from build123d import *

# Parameters (mm, degrees)
F1_DEPTH = 63.5
F2_DEPTH = 7.9375
F3_DEPTH = 25.4
F0_W     = 25.4
F0_H     = 28.575
F5_R     = 6.35


with BuildPart() as f1:
    # F0 (on Front) → F1 (new body, symmetric)
    with BuildSketch(Plane.XZ):
        Polygon((41.275, -9.525), (41.275, 9.525), (22.225, 9.525), (-41.275, 9.525), (-41.275, -9.525), align=None)
    extrude(amount=F1_DEPTH, both=True)

    # F0 (on Front) → F2 (join, symmetric)
    with BuildSketch(Plane.XZ):
        with BuildLine():
            Line((-41.275, 9.525), (22.225, 9.525))
            Line((22.225, 9.525), (22.225, 27.673652))
            ThreePointArc((22.225, 27.673652), (30.148747, 49.82513), (50.324526, 61.9252))
            add(Edge.make_bspline(
                [(-41.275, 9.525), (-34.773878, 42.640614), (12.253828, 61.712361), (50.324526, 61.9252)],
                knots=[0, 0, 0, 0, 105.528452, 105.528452, 105.528452, 105.528452], degree=3))
        make_face()
    extrude(amount=F2_DEPTH, both=True)

    # F0 (on Front) → F3 (join, symmetric)
    with BuildSketch(Plane.XZ):
        with BuildLine():
            Line((22.225, 9.525), (41.275, 9.525))
            Line((41.275, 9.525), (41.275, 27.673652))
            ThreePointArc((41.275, 27.673652), (47.109768, 39.970374), (60.325, 43.227912))
            Line((60.325, 43.227912), (60.325, 61.9252))
            Line((60.325, 61.9252), (50.324526, 61.9252))
            ThreePointArc((50.324526, 61.9252), (30.148747, 49.82513), (22.225, 27.673652))
            Line((22.225, 27.673652), (22.225, 9.525))
        make_face()
        with BuildLine():
            Line((60.325, 61.9252), (60.325, 43.227912))
            ThreePointArc((60.325, 43.227912), (61.028899, 43.067475), (61.724775, 42.8752))
            Line((61.724775, 42.8752), (68.150982, 42.8752))
            Line((68.150982, 42.8752), (68.150982, 61.9252))
            Line((68.150982, 61.9252), (60.325, 61.9252))
        make_face()
    extrude(amount=F3_DEPTH, both=True)

    # F0 (on Front) → F4 (revolve)
    with BuildSketch(Plane.XZ):
        with Locations((98.425, 52.3875)):
            Rectangle(F0_W, F0_H)
    revolve(axis=Axis((85.725, 0, 52.3875), (0, 0, -1)))

    # F5
    f5_edges = [f1.edges().sort_by_distance(p)[0] for p in [
        (41.275, -63.5, 0),
        (-41.275, -63.5, 0),
        (41.275, 63.5, 0),
        (-41.275, 63.5, 0),
    ]]
    fillet(f5_edges, radius=F5_R)


solid = f1.part
Read the model definition and answer for the solid it produces. Units are mm, in the model's axes. A direction names the side the tool comes from. Round coordinates to 2 decimals unless told otherwise and drop trailing zeros. Write each loop counter-clockwise with the first axis right and the second up, starting at its lowest first coordinate (ties: lowest second). Pieces come first, ordered by that corner, then holes.
Q1. A tool of negligible diameter and unlimited length cuts with its end or side. For faces 5 (the face through (30.36, 16.55, 50.08)), 6 (the face through (40, -25.4, 36)), 7 (the face through (86, 0, 38.1)), 8 (the face through (0, -63.5, 0)), 9 (the face through (-6, -7.938, 30)), from which of +Z, -Z, +X, -X, +Y, -Y can it reach the whole face along a straight path? Write none if from no direction.
Values:
face 5: +Z, -X, +Y
face 6: +Z, +X, -X, -Y
face 7: -Z, +X, +Y, -Y
face 8: +Z, -Z, +X, -X, -Y
face 9: +Z, -X, -Y
Q2. The mould has two halves that part along X. Classify faces 1 (the face through (39.464, -61.59, 0.133)), 2 (the face through (57, 0, 61.925)), 3 (the face through (64, 19, 42.875)), 4 (the face through (22.225, -17, 19)): released by +X, released by -X, zero draft, split by the parting line, or undercut.
Values:
face 1: released by +X
face 2: zero draft
face 3: undercut
face 4: released by -X
Q3. Flat-ended cylindrical pins translate along their axes: P1, Ø1.5, axis at x = -13, z = 43.5, coming from the -Y side; P2, Ø1, axis at y = -18.5, z = 49.5, coming from the -X side; P3, Ø2, axis at x = -18.5, y = -43.5, coming from the +Z side (3 decimals). Find the tip coordinate at first contact, or state that the pin passes through.
Values:
P1: stops at y = -7.94
P2: stops at x = 29.49
P3: stops at z = 9.525
Q4. Find section A-A on y = -28. Determine the outline of the cut face in (x, z) (3 decimals), and give its area (3 significant figures).
Values:
outline: (-41.275, -9.525) - (41.275, -9.525) - (41.275, 9.525) - (-41.275, 9.525) - close
area: 1,570 mm2
Q5. Straight lines are drawn through the part: line 1 (Y direction, x = 22, z = 25); line 2 (X direction, y = -50.5, z = 4) (3 decimals); line 3 (Y direction, x = 86, z = 57.5). For each, find the intervals that lie inside material, in ascending order.
Values:
line 1: y = -7.94 to 7.94
line 2: x = -41.275 to 41.275
line 3: y = -25.4 to 25.4
Q6. Find section B-B on x = 73.5. Determine the outline of the cut face in (y, z) (3 decimals).
Values:
outline: (-22.265, 38.1) - (22.265, 38.1) - (22.265, 66.675) - (-22.265, 66.675) - close
